from build123d import *

# Parameters (mm, degrees)
F0_R     = 9
F1_DEPTH = 160
F2_W     = 23.4179981053
F2_H     = 22.6416159421
F2_W_2   = 14.5
F2_H_2   = 13.2822632294
F3_DEPTH = 12
F4_R     = 10.315
F5_DEPTH = 25
F6_SIZE2 = 5.6712818196
F6_SIZE  = 1
F7_R     = 14.7612930143
F7_R_2   = 8
F8_DEPTH = 35


with BuildPart() as f1:
    # F0 (on Front) → F1 (new body)
    with BuildSketch(Plane.XZ):
        Circle(F0_R)
    extrude(amount=F1_DEPTH)

    # F2 (on face) → F3 (cut)
    with BuildSketch(Plane.XZ.offset(160)):
        Rectangle(F2_W, F2_H)
        Rectangle(F2_W_2, F2_H_2, mode=Mode.SUBTRACT)
    extrude(amount=-F3_DEPTH, mode=Mode.SUBTRACT)

    # F4 (on face) → F5 (join)
    with BuildSketch(Plane(origin=(0, 0, 0), x_dir=(-1, 0, 0), z_dir=(0, 1, 0))):
        Circle(F4_R)
    extrude(amount=-F5_DEPTH)

    # F6
    f6_edges = [f1.edges().sort_by_distance(p)[0] for p in [
        (10.315, 0, 0),
    ]]
    f6_side = f1.faces().sort_by_distance((0, 0, 0))[0]
    chamfer(f6_edges, length=F6_SIZE, length2=F6_SIZE2, reference=f6_side)

    # F7 (on face) → F8 (cut)
    with BuildSketch(Plane.XZ.offset(25)):
        Circle(F7_R)
        Circle(F7_R_2, mode=Mode.SUBTRACT)
    extrude(amount=F8_DEPTH, mode=Mode.SUBTRACT)


solid = f1.part
Could you check a few things on this model? Use its own coordinates, in mm. A direction names the side the tool comes from. Coordinates: 2 decimals unless noted, no trailing zeros. Order: outer loops, then holes, each group sorted by start corner. A loop starts at its lowest first (then second) coordinate and runs counter-clockwise, first axis right, second up. Notation, with made-up numbers: (29.25, -18.75) -> (64.25, -18.75) arc R17 ccw to (64.25, -6.75) -> close; hole circle Ø10 at (0.25, -39). An arc over 180 degrees is marked (long way). One line per item, written item: value. Start each with the question number.
1) I'm going to push flat-ended pins straight in: pin 1 (5.5 mm diameter, centred on y = -156.5, z = 0.5, fed in from +X); pin 2 (0.7 mm diameter, centred on x = -1.5, z = -7.5, fed in from -Y); pin 3 (12 mm diameter, centred on x = 5, y = -53, fed in from -Z). Where does each tip first touch, or does it pass through?
2) Which directions (+Z, -Z, +X, -X, +Y, -Y) give clear straight access to the entire face, cutting with the end or side of a thin tool? Please do faces 1 (the flat face through (7.25, -154, 0)), 2 (the cylindrical face through (-1.73, -42.26, -7.81)), 3 (the flat face through (0, -154, 6.641)), 4 (the flat face through (0, -154, -6.641)), 5 (the cylindrical face through (-9, -109, 0)).
3) Imagine slicing it at A-A on x = 0. List the corners of the cut face in (y, z) for me (3 decimals), plus the area to 3 significant figures.
4) Imagine slicing it at C-C on y = -82. List the corners of the cut face in (x, z) for me.
5) If I drill on L1, parallel to Y at x = 3.5, z = -8; L2, parallel to Y at x = 1.75, z = 7.25; L3, parallel to Y at x = -7.25, z = -5.5, over which ranges is the centre line in solid material (lowest first)? Write a range as [from, to].
6) Imagine slicing it at B-B on z = 0. List the corners of the cut face in (x, y) for me (3 decimals), plus the area to 3 significant figures.
Answer list:
1. pin 1: stops at x = 7.25
1. pin 2: stops at y = -148
1. pin 3: stops at z = -8
2. face 1: +Z, -Z, +X, -Y
2. face 2: none
2. face 3: +Z, +X, -X, -Y
2. face 4: -Z, +X, -X, -Y
2. face 5: -Y
3. outline: (-160, -6.641) -> (-148, -6.641) -> (-148, -9) -> (-60, -9) -> (-60, -8) -> (-25, -8) -> (-25, -10.315) -> (-5.671, -10.315) -> (0, -9.315) -> (0, 9.315) -> (-5.671, 10.315) -> (-25, 10.315) -> (-25, 8) -> (-60, 8) -> (-60, 9) -> (-148, 9) -> (-148, 6.641) -> (-160, 6.641) -> close
3. area: 2,810 mm2
4. outline: circle Ø18 at (0, 0)
5. L1: y = [-148, -60], [-25, 0]
5. L2: y = [-148, 0]
5. L3: y = [-25, 0]
6. outline: (-10.315, -25) -> (-8, -25) -> (-8, -60) -> (-9, -60) -> (-9, -148) -> (-7.25, -148) -> (-7.25, -160) -> (7.25, -160) -> (7.25, -148) -> (9, -148) -> (9, -60) -> (8, -60) -> (8, -25) -> (10.315, -25) -> (10.315, -5.671) -> (9.315, 0) -> (-9.315, 0) -> (-10.315, -5.671) -> close
6. area: 2,830 mm2
